Verification items for this drawing (mm, ordinates from the low corner). A direction names the side the tool comes from. Coordinates: 2 decimals unless noted, no trailing zeros. Loops run counter-clockwise (first coordinate to the right, second up) from the corner with the lowest first, then second, coordinate; pieces in that order, holes last. Notation, with made-up numbers: (80, 35.25) - (111, 35.25) arc R16 cw to (111, 40.25) - close; hole circle Ø9 at (82.5, 21.25). An arc over 180 degrees is marked (long way). One line per item, written item: value. Start each with the question number.
(1) Set-up check for the marked faces 1, 2 and 3: record each of +Z, -Z, +X, -X, +Y, -Y from which the full face is reachable in a straight line by a thin tool's end or side.
(2) Thickness scan on probe 1 along Y at (x, z) = (19.5, 66.5) (1 decimal); probe 2 along Z at (x, y) = (16.5, 7); probe 3 along Z at (x, y) = (24, 15.5). Record the ranges inside material, lowest first. Write a range as [from, to].
(3) Gauge pin test, flat ends, axial feed: P1, Ø1, axis at y = 21, z = 68.5, coming from the +X side; P2, Ø3.5, axis at x = 5.5, y = 10, coming from the +Z side; P3, Ø2.5, axis at x = 31.82, y = 10.65, coming from the +Z side. Record the tip position at first contact, or that the pin passes through.
(4) Section check D-D (y = 18.4). Record the boundary of the cut face in (x, z).
(5) Section check B-B (y = 31). Record the boundary of the cut face in (x, z), plus the area to 4 significant figures.
(6) Section check C-C (z = 60). Record the boundary of the cut face in (x, y), plus the area to 3 significant figures.
(7) Section check A-A (x = 18.4). Record the boundary of the cut face in (y, z), plus the area to 3 significant figures.
(8) Draft check along Y on the marked faces 4 and 5. Enter one of: +Y half, -Y half, draft (parallel to the pull), parting line (faces both ways), or undercut.
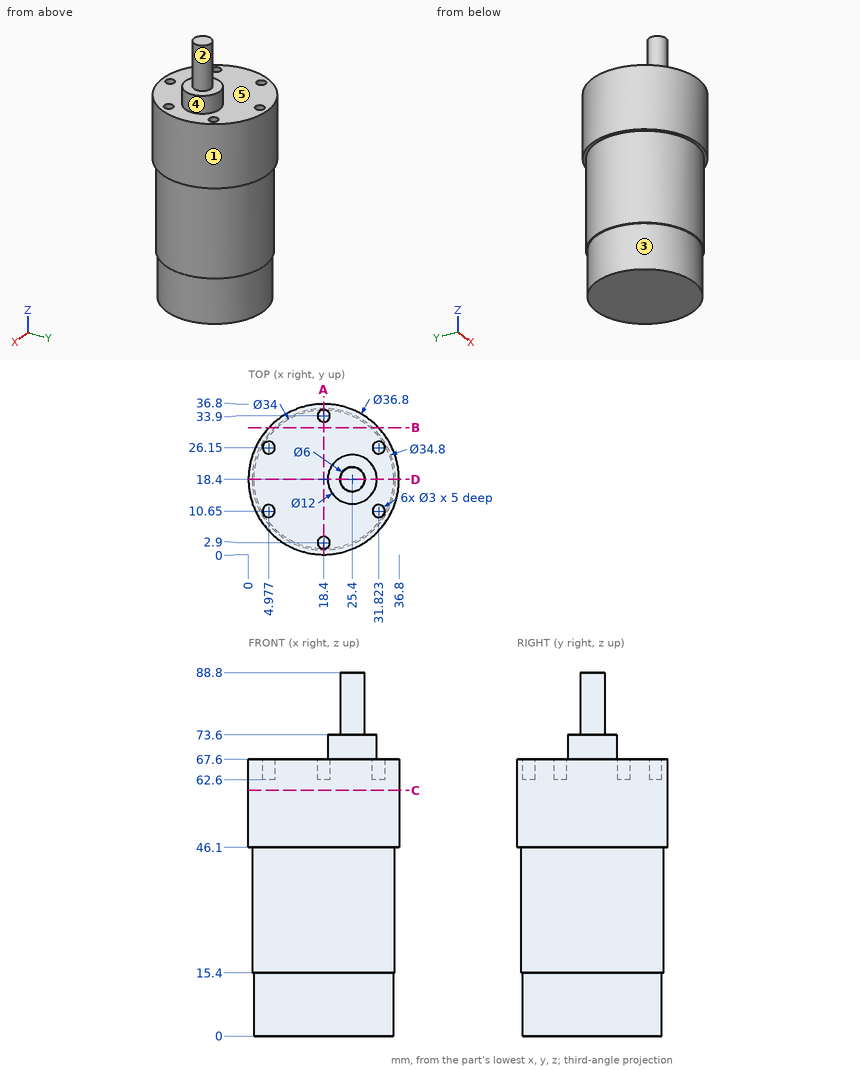
Responses:
1. face 1: +Z, -Z
1. face 2: +Z
1. face 3: -Z
2. probe 1: y = [0, 1.9], [3.9, 32.9], [34.9, 36.8]
2. probe 2: z = [0, 67.6]
2. probe 3: z = [0, 73.6]
3. P1: stops at x = 31.02
3. P2: stops at z = 67.6
3. P3: stops at z = 62.6
4. outline: (0, 46.1) - (1, 46.1) - (1, 15.4) - (1.4, 15.4) - (1.4, 0) - (35.4, 0) - (35.4, 15.4) - (35.8, 15.4) - (35.8, 46.1) - (36.8, 46.1) - (36.8, 67.6) - (31.4, 67.6) - (31.4, 73.6) - (28.4, 73.6) - (28.4, 88.8) - (22.4, 88.8) - (22.4, 73.6) - (19.4, 73.6) - (19.4, 67.6) - (0, 67.6) - close
5. outline: (4.99, 46.1) - (6.4, 46.1) - (6.4, 15.4) - (6.99, 15.4) - (6.99, 0) - (29.81, 0) - (29.81, 15.4) - (30.4, 15.4) - (30.4, 46.1) - (31.81, 46.1) - (31.81, 67.6) - (4.99, 67.6) - close
5. area: 1,665 mm²
6. outline: circle Ø36.8 at (18.4, 18.4)
6. area: 1,060 mm²
7. outline: (0, 46.1) - (1, 46.1) - (1, 15.4) - (1.4, 15.4) - (1.4, 0) - (35.4, 0) - (35.4, 15.4) - (35.8, 15.4) - (35.8, 46.1) - (36.8, 46.1) - (36.8, 67.6) - (35.4, 67.6) - (35.4, 62.6) - (32.4, 62.6) - (32.4, 67.6) - (4.4, 67.6) - (4.4, 62.6) - (1.4, 62.6) - (1.4, 67.6) - (0, 67.6) - close
7. area: 2,350 mm²
8. face 4: parting line
8. face 5: draft
